Read the model definition and answer for the solid it produces. Units are mm, in the model's axes. Face numbers are marked on the shaded views. A direction names the side the tool comes from. Coordinates: 2 decimals unless noted, no trailing zeros. Write each loop counter-clockwise with the first axis right and the second up, starting at its lowest first coordinate (ties: lowest second). Pieces come first, ordered by that corner, then holes.
1) The part is cut by section C-C (z = -8). Determine the outline of the cut face in (x, y).
2) Each of these flat-tipped pins is pushed along its axis until it touches: pin 1 Ø6 at (x, y) = (0, 0) entering from -Z; pin 2 Ø6 at (x, z) = (8, -8) entering from +Y; pin 3 Ø1 at (x, z) = (6, -4.5) entering from -Y; pin 4 Ø1 at (x, z) = (-8, -3.5) entering from +Y. Where does it stop, or does it pass through?
3) Determine the mould class of the marked faces 1, 2 and 3 for opening direction X: +X half, -X half, draft (parallel to the pull), parting line (faces both ways), or undercut.
4) The part is cut by section A-A (x = 0). Determine the outline of the cut face in (y, z), then the cut area to 3 significant figures.
5) Find the intervals of material crossed by line 1 (Z direction, x = -2.75, y = 3.5); line 2 (X direction, y = -2.5, z = -4); line 3 (Y direction, x = -2.5, z = -1.5), in increasing order.
6) The part is cut by section D-D (z = -10). Determine the outline of the cut face in (x, y), then the cut area to 3 significant figures.
7) Which of the six approach directions +Z, -Z, +X, -X, +Y, -Y give full straight-line access (tool end or side, diameter ignored) to the marked faces 4 and 5?
from build123d import *

# Parameters (mm, degrees)
ENL_V_MAT_EXTRU_1_REACH = 23.366
ESQUISSE2_R             = 2.25
ESQUISSE3_R             = 5
ENL_V_MAT_EXTRU_2_DEPTH = 5
CONG_1_R                = 2


with BuildPart() as part:
    # Esquisse1 → Révolution1 (revolve)
    with BuildSketch(Plane(origin=(0, 0, 0), x_dir=(0, 0, -1), z_dir=(1, 0, 0)), mode=Mode.PRIVATE) as r_volution1_sk:
        Polygon((0, 0), (12, 0), (12, 12.5), (0, 10), align=None)
    revolve(r_volution1_sk.sketch.rotate(Axis((0, 0, 0), (0, 0, -1)), 90), axis=Axis((0, 0, 0), (0, 0, -1)))

    # Esquisse2 → Enlèv. mat.-Extru.1 (cut, up to next)
    with BuildSketch(Plane.XY, mode=Mode.PRIVATE) as enl_v_mat_extru_1_sk1:
        Circle(ESQUISSE2_R)
    enl_v_mat_extru_1_tool1 = extrude(enl_v_mat_extru_1_sk1.sketch, amount=-ENL_V_MAT_EXTRU_1_REACH, mode=Mode.PRIVATE) & part.part
    add(enl_v_mat_extru_1_tool1.solids().sort_by_distance((0, 0, 0))[0], mode=Mode.SUBTRACT)

    # Esquisse3 → Enlèv. mat.-Extru.2 (cut)
    with BuildSketch(Plane.XY):
        Circle(ESQUISSE3_R)
    extrude(amount=-ENL_V_MAT_EXTRU_2_DEPTH, mode=Mode.SUBTRACT)

    # Congé1
    cong_1_edges = [part.edges().sort_by_distance(p)[0] for p in [
        (-5, 0, 0),
        (-10, 0, 0),
    ]]
    fillet(cong_1_edges, radius=CONG_1_R)


solid = part.part
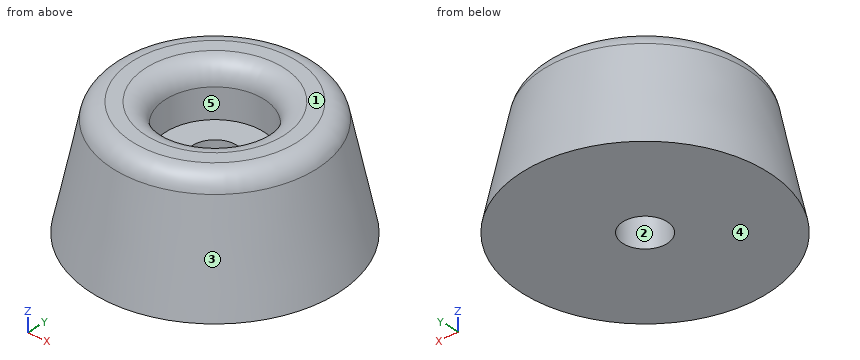
Reported:
1. outline: circle Ø23.33 at (0, 0); hole circle Ø4.5 at (0, 0)
2. pin 1: stops at z = -12
2. pin 2: stops at y = 10.7
2. pin 3: stops at y = -9.48
2. pin 4: stops at y = 7.69
3. face 1: draft
3. face 2: undercut
3. face 3: parting line
4. outline: (-12.5, -12) - (-2.25, -12) - (-2.25, -5) - (-5, -5) - (-5, -2) arc R2 ccw to (-7, 0) - (-8.37, 0) arc R2 ccw to (-10.33, -1.59) - close; (2.25, -12) - (12.5, -12) - (10.33, -1.59) arc R2 ccw to (8.37, 0) - (7, 0) arc R2 ccw to (5, -2) - (5, -5) - (2.25, -5) - close
4. area: 186 mm2
5. line 1: z = -12 to -5
5. line 2: x = -10.54 to -4.33, 4.33 to 10.54
5. line 3: y = -10 to -4.4, 4.4 to 10
6. outline: circle Ø24.17 at (0, 0); hole circle Ø4.5 at (0, 0)
6. area: 443 mm2
7. face 4: -Z, +X, -X, +Y, -Y
7. face 5: +Z
